Input: part model. Units: mm. Frame: model coordinates. Coordinates: 2 decimals unless noted, no trailing zeros. Loops run counter-clockwise (first coordinate to the right, second up) from the corner with the lowest first, then second, coordinate; pieces in that order, holes last.
```python
from build123d import *

# Parameters (mm, degrees)
EXTRUSION1_DEPTH          = 282
TROU_TARAUD_M4X0_72_D     = 3.3
TROU_TARAUD_M4X0_72_DEPTH = 17.1
TROU_TARAUD_M4X0_72_TIP   = 0.991420021
TROU_TARAUD_M4X0_73_D     = 3.3
TROU_TARAUD_M4X0_73_DEPTH = 9.1
TROU_TARAUD_M4X0_73_TIP   = 0.991420021
TROU_TARAUD_M4X0_74_D     = 3.3
TROU_TARAUD_M4X0_75_D     = 3.3
TROU_TARAUD_M4X0_76_D     = 3.3


with BuildPart() as part:
    # Esquisse1 → Extrusion1 (new body)
    with BuildSketch(Plane(origin=(0, 0, 0), x_dir=(1, 0, 0), z_dir=(0, 1, 0))):
        with BuildLine():
            Line((0.353553391, 10.253048327), (10.253048327, 0.353553391))
            ThreePointArc((10.253048327, 0.353553391), (10.399494937, 0), (10.253048327, -0.353553391))
            Line((10.253048327, -0.353553391), (0.353553391, -10.253048327))
            ThreePointArc((0.353553391, -10.253048327), (0, -10.399494937), (-0.353553391, -10.253048327))
            Line((-0.353553391, -10.253048327), (-10.253048327, -0.353553391))
            ThreePointArc((-10.253048327, -0.353553391), (-10.399494937, 0), (-10.253048327, 0.353553391))
            Line((-10.253048327, 0.353553391), (-0.353553391, 10.253048327))
            ThreePointArc((-0.353553391, 10.253048327), (0, 10.399494937), (0.353553391, 10.253048327))
        make_face()
    extrude(amount=EXTRUSION1_DEPTH)

    # Trou taraudé M4x0.72
    with Locations(Plane.XZ):
        with Locations((0, 0)):
            Hole(TROU_TARAUD_M4X0_72_D / 2, depth=TROU_TARAUD_M4X0_72_DEPTH)
            with Locations((0, 0, -(TROU_TARAUD_M4X0_72_DEPTH + TROU_TARAUD_M4X0_72_TIP / 2))):  # 118° drill point
                Cone(0, TROU_TARAUD_M4X0_72_D / 2, TROU_TARAUD_M4X0_72_TIP, mode=Mode.SUBTRACT)

    # Trou taraudé M4x0.73
    with Locations(Plane(origin=(0, 282, 0), x_dir=(-1, 0, 0), z_dir=(0, 1, 0))):
        with Locations((0, 0)):
            Hole(TROU_TARAUD_M4X0_73_D / 2, depth=TROU_TARAUD_M4X0_73_DEPTH)
            with Locations((0, 0, -(TROU_TARAUD_M4X0_73_DEPTH + TROU_TARAUD_M4X0_73_TIP / 2))):  # 118° drill point
                Cone(0, TROU_TARAUD_M4X0_73_D / 2, TROU_TARAUD_M4X0_73_TIP, mode=Mode.SUBTRACT)

    # Trou taraudé M4x0.74 (through all)
    with Locations(Plane(origin=(-5.303300859, 0, 5.303300859), x_dir=(0.7071067811865477, 0, 0.7071067811865474), z_dir=(-0.7071067811865474, 0, 0.7071067811865477))):
        with Locations((0, 91), (0, 32)):
            Hole(TROU_TARAUD_M4X0_74_D / 2)

    # Trou taraudé M4x0.75 (through all)
    with Locations(Plane(origin=(-5.303300859, 0, -5.303300859), x_dir=(-0.7071067811865477, 0, 0.7071067811865475), z_dir=(-0.7071067811865475, 0, -0.7071067811865477))):
        with Locations((0, 98.5), (0, 247)):
            Hole(TROU_TARAUD_M4X0_75_D / 2)

    # Trou taraudé M4x0.76 (through all)
    with Locations(Plane(origin=(5.303300859, 0, -5.303300859), x_dir=(-0.7071067811865474, 0, -0.7071067811865477), z_dir=(0.7071067811865477, 0, -0.7071067811865474))):
        with Locations((0, 268.6), (0, 252.6)):
            Hole(TROU_TARAUD_M4X0_76_D / 2)


solid = part.part
```
Item 1: Mould query, pull axis Z, two halves, no side actions, for faces 1 (the face through (5.234, 139.026, -5.373)), 2 (the face through (-5.234, 139.026, 5.373)), 3 (the face through (-0.18, 96.89, 0.33)), 4 (the face through (0.226, 33.636, 0.078)). Classes: +Z half, -Z half, draft (parallel to the pull), parting line (faces both ways), or undercut.
Result:
face 1: -Z half
face 2: +Z half
face 3: undercut
face 4: undercut
Item 2: Section query A-A (y = 211). Output: boundary loops of the cut face in (x, z).
Result:
outline: (-10.25, -0.35) - (-0.35, -10.25) arc R0.5 ccw to (0.35, -10.25) - (10.25, -0.35) arc R0.5 ccw to (10.25, 0.35) - (0.35, 10.25) arc R0.5 ccw to (-0.35, 10.25) - (-10.25, 0.35) arc R0.5 ccw to start
Item 3: Line query: L1, parallel to Z at x = 0, y = 13; L2, parallel to Y at x = -2, z = -1. Output: solid intervals per line, ascending.
Result:
L1: z = -10.4 to -1.65, 1.65 to 10.4
L2: y = 0 to 97.01, 99.99 to 245.51, 248.49 to 282
Item 4: Contact query for flat-ended pins moving along their axis: P1, Ø3, axis at x = -2.5, y = 72, coming from the +Z side; P2, Ø3, axis at y = 169, z = 4, coming from the -X side; P3, Ø1.5, axis at x = 4, y = 64, coming from the +Z side. Output: stop coordinate, or through.
Result:
P1: stops at z = 9.61
P2: stops at x = -8.11
P3: stops at z = 7.36
